Work out the finished part from the listing and answer in its coordinate system (mm). Face numbers are marked on the shaded views. A direction names the side the tool comes from. Coordinates: 2 decimals unless noted, no trailing zeros. Order: outer loops, then holes, each group sorted by start corner. A loop starts at its lowest first (then second) coordinate and runs counter-clockwise, first axis right, second up. Notation, with made-up numbers: (1, -10.5) - (12, -10.5) arc R29 cw to (12, 16.5) - close; hole circle Ø11 at (37, -11). An arc over 180 degrees is marked (long way). Answer as a JSON object with one key per item and string values. Group by question number.
1) Section B-B (x = 0) is taken. Give the vertices of the cut face in (y, z), plus the area to 3 significant figures.
2) Section C-C (y = 2.25) is taken. Give the vertices of the cut face in (x, z).
3) The mould has two halves that part along X. Classify the marked faces 1, 2 and 3: released by +X, released by -X, zero draft, split by the parting line, or undercut.
4) A tool of negligible diameter and unlimited length cuts with its end or side. For the marked faces 4, 5 and 6, from which of +Z, -Z, +X, -X, +Y, -Y can it reach the whole face along a straight path? Write none if from no direction.
5) This flat-tipped pin is pushed along its axis until it touches: P1, Ø1.5, axis at x = -3, y = 1.5, coming from the +Z side. Where does it stop, or does it pass through?
6) Find the intervals of material crossed by line 1 along Z through (x, y) = (0, 1.15); line 2 along Y through (x, z) = (1.25, 0.25); line 3 along Y through (x, z) = (-2, 3.5), in increasing order.
7) Section A-A (z = 0) is taken. Give the vertices of the cut face in (x, y) (3 decimals).
8) Section D-D (y = 4.25) is taken. Give the vertices of the cut face in (x, z).
from build123d import *

# Parameters (mm, degrees)
SKETCH1_R           = 3.25
BOSS_EXTRUDE1_DEPTH = 2.46
SKETCH2_R           = 1.75
CUT_EXTRUDE1_DEPTH  = 2.5
SKETCH6_R           = 4.8
BOSS_EXTRUDE2_DEPTH = 5
FILLET2_R           = 0.75
SKETCH7_R           = 1.5
BOSS_EXTRUDE3_DEPTH = 1


with BuildPart() as part:
    # Sketch1 → Boss-Extrude1 (new body)
    with BuildSketch(Plane(origin=(0, 0, 0), x_dir=(1, 0, 0), z_dir=(0, 1, 0))):
        Circle(SKETCH1_R)
    extrude(amount=BOSS_EXTRUDE1_DEPTH)

    # Sketch2 → Cut-Extrude1 (cut)
    with BuildSketch(Plane.XZ):
        Circle(SKETCH2_R)
    extrude(amount=-CUT_EXTRUDE1_DEPTH, mode=Mode.SUBTRACT)

    # Sketch6 → Boss-Extrude2 (add)
    with BuildSketch(Plane(origin=(0, 2.46, 0), x_dir=(1, 0, 0), z_dir=(0, 1, 0))):
        Circle(SKETCH6_R)
    extrude(amount=BOSS_EXTRUDE2_DEPTH)

    # Fillet2
    fillet2_edges = [part.edges().sort_by_distance(p)[0] for p in [
        (-4.8, 7.46, 0),
    ]]
    fillet(fillet2_edges, radius=FILLET2_R)

    # Sketch7 → Boss-Extrude3 (add)
    with BuildSketch(Plane(origin=(0, 7.46, 0), x_dir=(1, 0, 0), z_dir=(0, 1, 0))):
        with Locations((-2.025, 0)):
            Circle(SKETCH7_R)
        with Locations((2.025, 0)):
            Circle(SKETCH7_R)
    extrude(amount=BOSS_EXTRUDE3_DEPTH)


solid = part.part
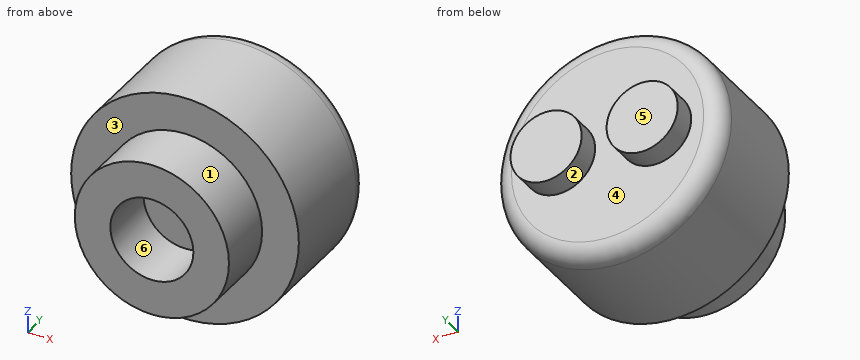
Report:
{
 "1": {"outline": "(0, -3.25) - (2.46, -3.25) - (2.46, -4.8) - (6.71, -4.8) arc R0.75 ccw to (7.46, -4.05) - (7.46, 4.05) arc R0.75 ccw to (6.71, 4.8) - (2.46, 4.8) - (2.46, 3.25) - (0, 3.25) - (0, 1.75) - (2.46, 1.75) - (2.46, -1.75) - (0, -1.75) - close", "area": "55.1 mm²"},
 "2": {"outline": "circle Ø6.5 at (0, 0); hole circle Ø3.5 at (0, 0)"},
 "3": {"face 1": "split by the parting line", "face 2": "undercut", "face 3": "zero draft"},
 "4": {"face 4": "+Y", "face 5": "+Z, -Z, +X, -X, +Y", "face 6": "-Y"},
 "5": {"P1": "stops at z = 2.35"},
 "6": {"line 1": "z = -3.25 to -1.75, 1.75 to 3.25", "line 2": "y = 2.46 to 8.46", "line 3": "y = 2.46 to 7.46"},
 "7": {"outline": "(-4.8, 2.46) - (-3.25, 2.46) - (-3.25, 0) - (-1.75, 0) - (-1.75, 2.46) - (1.75, 2.46) - (1.75, 0) - (3.25, 0) - (3.25, 2.46) - (4.8, 2.46) - (4.8, 6.71) arc R0.75 ccw to (4.05, 7.46) - (3.525, 7.46) - (3.525, 8.46) - (0.525, 8.46) - (0.525, 7.46) - (-0.525, 7.46) - (-0.525, 8.46) - (-3.525, 8.46) - (-3.525, 7.46) - (-4.05, 7.46) arc R0.75 ccw to (-4.8, 6.71) - close"},
 "8": {"outline": "circle Ø9.6 at (0, 0)"}
}
